Read the model definition and answer for the solid it produces. Units are mm, in the model's axes. A direction names the side the tool comes from. Give positions to 0.01 mm unless a question says otherwise; leave off trailing zeros. Write each loop counter-clockwise with the first axis right and the second up, starting at its lowest first coordinate (ties: lowest second). Pieces come first, ordered by that corner, then holes.
```python
from build123d import *

# Parameters (mm, degrees)
BOSS_EXTRUDE1_DEPTH     = 246
CUT_EXTRUDE1_DEPTH      = 78
BOSS_EXTRUDE2_START     = 33
BOSS_EXTRUDE2_DEPTH     = 33
CUT_EXTRUDE4_DEPTH      = 13
CUT_EXTRUDE5_REACH      = 314.807
CUT_EXTRUDE5_END_RADIUS = 28.575


with BuildPart() as part:
    # Sketch2 → Boss-Extrude1 (new body)
    with BuildSketch(Plane.XY):
        with BuildLine():
            Line((0, -28.575), (0, -84))
            Line((0, -84), (-13, -84))
            Line((-13, -84), (-84, -43.008130888))
            Line((-84, -43.008130888), (-84, 0))
            ThreePointArc((-84, 0), (-59.39696962, 59.39696962), (0, 84))
            Line((0, 84), (0, 28.575))
            ThreePointArc((0, 28.575), (-28.575, 0), (0, -28.575))
        make_face()
    extrude(amount=-BOSS_EXTRUDE1_DEPTH)

    # Sketch3 → Cut-Extrude1 (cut)
    with BuildSketch(Plane.XY):
        with BuildLine():
            Line((0, 44.45), (0, 28.575))
            ThreePointArc((0, 28.575), (-28.575, 0), (0, -28.575))
            Line((0, -28.575), (0, -44.45))
            ThreePointArc((0, -44.45), (-44.45, 0), (0, 44.45))
        make_face()
    extrude(amount=-CUT_EXTRUDE1_DEPTH, mode=Mode.SUBTRACT)

    # Sketch4 → Boss-Extrude2 (add)
    with BuildSketch(Plane.XY.offset(BOSS_EXTRUDE2_START)):
        with BuildLine():
            Line((-20.856290899, 81.369620436), (-8.61759969, 71.807706907))
            Line((-8.61759969, 71.807706907), (-59.101840666, 7.190825111))
            Line((-59.101840666, 7.190825111), (-80.520739305, 23.925102753))
            ThreePointArc((-80.520739305, 23.925102753), (-58.260567421, 60.512034206), (-20.856290899, 81.369620436))
        make_face()
    extrude(amount=-BOSS_EXTRUDE2_DEPTH)

    # Sketch8 → Cut-Extrude4 (cut)
    with BuildSketch(Plane(origin=(0, 0, 0), x_dir=(0, 0, -1), z_dir=(1, 0, 0))):
        with BuildLine():
            Line((246, -47), (129, -47))
            ThreePointArc((129, -47), (118, -58), (129, -69))
            Line((129, -69), (246, -69))
            Line((246, -69), (246, -47))
        make_face()
    extrude(amount=-CUT_EXTRUDE4_DEPTH, mode=Mode.SUBTRACT)

    # Cut-Extrude5: up to this cylinder (the profile starts outside it)
    cut_extrude5_end = Plane(origin=(0, 0, -191.5), z_dir=(0, 0, 1)) * Cylinder(CUT_EXTRUDE5_END_RADIUS, 687.764, mode=Mode.PRIVATE)
    # Sketch9 → Cut-Extrude5 (cut, up to the surface)
    with BuildSketch(Plane(origin=(0, 90, 0), x_dir=(1, 0, 0), z_dir=(0, 1, 0)), mode=Mode.PRIVATE) as cut_extrude5_sk1:
        Polygon((0, 175), (0, 208), (-19, 206.337715393), (-19, 176.662284607), align=None)
    cut_extrude5_tool1 = extrude(cut_extrude5_sk1.sketch, amount=-CUT_EXTRUDE5_REACH, mode=Mode.PRIVATE) - cut_extrude5_end
    add(cut_extrude5_tool1.solids().sort_by_distance((-9.332027, 90, -191.5))[0], mode=Mode.SUBTRACT)


solid = part.part
```
Item 1: Each of these flat-tipped pins is pushed along its axis until it touches: pin 1 Ø22 at (x, y) = (-18.5, 20.5) entering from +Z; pin 2 Ø9 at (y, z) = (44.5, -191) entering from +X; pin 3 Ø4 at (x, z) = (-4.5, -179.5) entering from +Y. Where does it stop, or does it pass through?
Result set:
pin 1: stops at z = -78
pin 2: stops at x = -19
pin 3: stops at y = -27.83
Item 2: Determine the mould class of faces 6 (the flat face through (-44, 45, 33)), 7 (the flat face through (-19, 52, -192)), 8 (the flat face through (-6, -69, -187)) for opening direction Z: pulls with the +Z half, pulls with the -Z half, needs draft (parallel to the pull), parting line crosses it, or undercut.
Result set:
face 6: pulls with the +Z half
face 7: undercut
face 8: needs draft
Item 3: Which of the six approach directions +Z, -Z, +X, -X, +Y, -Y give full straight-line access (tool end or side, diameter ignored) to faces 1 (the flat face through (-9.37, 53.11, -207.18)), 2 (the cylindrical face through (-6, -58, -118)), 3 (the cylindrical face through (-44.44, -0.98, -38.45)), 4 (the flat face through (-69.66, 15.44, 16.73)), 5 (the flat face through (-14.823, 76.656, 16.731))?
Result set:
face 1: +X, +Y
face 2: -Z, +X
face 3: +Z, +X
face 4: +Z, -X, -Y
face 5: +Z, +X, +Y
Item 4: Find the intervals of material crossed by line 1 along Y through (x, z) = (-4.5, -122.5); line 2 along Y through (x, z) = (-23, -162.5); line 3 along Z through (x, y) = (-24, -56.5), in increasing order.
Result set:
line 1: y = -84 to -66.87, -49.13 to -28.22, 28.22 to 83.88
line 2: y = -78.23 to -16.96, 16.96 to 80.79
line 3: z = -246 to 0
Item 5: Section D-D (z = -172) is taken. Write down the section's boundary in (x, y) (3 decimals), and give its area (3 significant figures).
Result set:
outline: (-84, -43.008) - (-13, -84) - (0, -84) - (0, -69) - (-13, -69) - (-13, -47) - (0, -47) - (0, -28.575) arc R28.575 cw to (0, 28.575) - (0, 84) arc R84 ccw to (-84, 0) - close
area: 9,570 mm2
Item 6: Section B-B (x = -50.5) is taken. Write down the section's boundary in (y, z).
Result set:
outline: (-62.35, -246) - (67.12, -246) - (67.12, 33) - (18.2, 33) - (18.2, 0) - (-62.35, 0) - close
Item 7: Section C-C (y = 16) is taken. Write down the section's boundary in (x, z), and give its area (3 significant figures).
Result set:
outline: (-82.46, -246) - (-23.68, -246) - (-23.68, -78) - (-41.47, -78) - (-41.47, 0) - (-52.22, 0) - (-52.22, 33) - (-70.38, 33) - (-70.38, 0) - (-82.46, 0) - close
area: 13,700 mm2
Item 8: Section A-A (z = -8) is taken. Write down the section's boundary in (x, y), and give its area (3 significant figures).
Result set:
outline: (-84, -43.01) - (-13, -84) - (0, -84) - (0, -44.45) arc R44.45 cw to (0, 44.45) - (0, 84) arc R84 ccw to (-84, 0) - close
area: 8,040 mm2
